from build123d import *

# Parameters (mm, degrees)
ESQUISSE1_W        = 42.5
ESQUISSE1_H        = 45.220937172
BOSS_EXTRU_1_DEPTH = 50
ESQUISSE2_R        = 2.5
BOSS_EXTRU_2_DEPTH = 30
CONG_1_R           = 5
CONG_2_R           = 1
CONG_3_R           = 1


with BuildPart() as part:
    # Esquisse1 → Boss.-Extru.1 (new body)
    with BuildSketch(Plane.XY):
        Rectangle(ESQUISSE1_W, ESQUISSE1_H)
    extrude(amount=BOSS_EXTRU_1_DEPTH)

    # Esquisse2 → Boss.-Extru.2 (add)
    with BuildSketch(Plane(origin=(0, 0, 0), x_dir=(-1, 0, 0), z_dir=(0, 0, -1))):
        Circle(ESQUISSE2_R)
    extrude(amount=BOSS_EXTRU_2_DEPTH)

    # Congé1
    cong_1_edges = [part.edges().sort_by_distance(p)[0] for p in [
        (21.25, -22.610468586, 25),
        (-21.25, -22.610468586, 25),
        (-21.25, 22.610468586, 25),
        (21.25, 22.610468586, 25),
    ]]
    fillet(cong_1_edges, radius=CONG_1_R)

    # Congé2
    cong_2_edges = [part.edges().sort_by_distance(p)[0] for p in [
        (-21.25, 0, 50),
        (0, 22.610468586, 50),
        (21.25, 0, 50),
        (0, -22.610468586, 50),
        (19.785533906, 21.146002492, 50),
        (19.785533906, -21.146002492, 50),
        (-19.785533906, -21.146002492, 50),
        (-19.785533906, 21.146002492, 50),
    ]]
    fillet(cong_2_edges, radius=CONG_2_R)

    # Congé3
    cong_3_edges = [part.edges().sort_by_distance(p)[0] for p in [
        (-21.25, 0, 0),
        (21.25, 0, 0),
        (0, -22.610468586, 0),
        (0, 22.610468586, 0),
        (19.785533906, 21.146002492, 0),
        (19.785533906, -21.146002492, 0),
        (-19.785533906, -21.146002492, 0),
        (-19.785533906, 21.146002492, 0),
    ]]
    fillet(cong_3_edges, radius=CONG_3_R)


solid = part.part
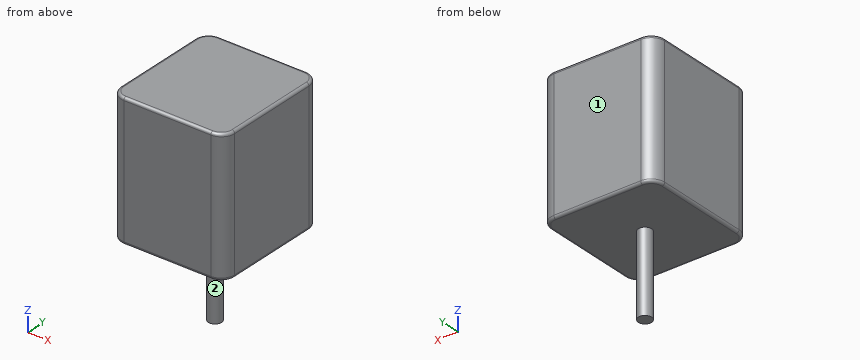
Here's how the part is built. I have some questions about the finished solid (model axes, mm). Face numbers are marked on the shaded views. A direction names the side the tool comes from. Round coordinates to 2 decimals unless told otherwise and drop trailing zeros. Write each loop counter-clockwise with the first axis right and the second up, starting at its lowest first coordinate (ties: lowest second). Pieces come first, ordered by that corner, then holes.
1. Suppose I cut it at D-D (y = -10.5). List the corners of the cut face in (x, z) for me.
2. For the marked faces 1 and 2, which set-ups out of +Z, -Z, +X, -X, +Y, -Y let a thin tool reach every point of the face, with its end or its side?
3. I need wall thicknesses on L1, parallel to Z at x = -18.5, y = 15.5; L2, parallel to X at y = 1, z = -22. Which ranges of each line are inside material? Lowest first, please.
4. Will these pins go through, and if not, where does the flat tip stop? pin 1 Ø12 at (x, z) = (-6.5, -10.5) entering from -Y; pin 2 Ø10 at (y, z) = (-1.5, -10.5) entering from -X.
5. Suppose I cut it at A-A (x = 0). List the corners of the cut face in (y, z) for me.
6. Suppose I cut it at B-B (y = 0). List the corners of the cut face in (x, z) for me.
7. Suppose I cut it at C-C (z = -14). List the corners of the cut face in (x, y) for me.
Answer sheet:
1. outline: (-21.25, 1) arc R1 ccw to (-20.25, 0) - (20.25, 0) arc R1 ccw to (21.25, 1) - (21.25, 49) arc R1 ccw to (20.25, 50) - (-20.25, 50) arc R1 ccw to (-21.25, 49) - close
2. face 1: +Z, -Z, +X, -X, +Y
2. face 2: -Z
3. L1: z = 0 to 50
3. L2: x = -2.29 to 2.29
4. pin 1: stops at y = -2.45
4. pin 2: stops at x = -2.5
5. outline: (-22.61, 1) arc R1 ccw to (-21.61, 0) - (-2.5, 0) - (-2.5, -30) - (2.5, -30) - (2.5, 0) - (21.61, 0) arc R1 ccw to (22.61, 1) - (22.61, 49) arc R1 ccw to (21.61, 50) - (-21.61, 50) arc R1 ccw to (-22.61, 49) - close
6. outline: (-21.25, 1) arc R1 ccw to (-20.25, 0) - (-2.5, 0) - (-2.5, -30) - (2.5, -30) - (2.5, 0) - (20.25, 0) arc R1 ccw to (21.25, 1) - (21.25, 49) arc R1 ccw to (20.25, 50) - (-20.25, 50) arc R1 ccw to (-21.25, 49) - close
7. outline: circle Ø5 at (0, 0)
